The model under review builds one solid part; all positions refer to its coordinate system, in mm. Coordinates: 2 decimals unless noted, no trailing zeros. Write each loop counter-clockwise with the first axis right and the second up, starting at its lowest first coordinate (ties: lowest second). Pieces come first, ordered by that corner, then holes. Notation, with made-up numbers: (62, 21) - (91, 21) arc R13 ccw to (91, 43) - close; hole circle Ø10 at (-36, 63). An arc over 180 degrees is marked (long way). Put each result on its own line as item: value.
from build123d import *

# Parameters (mm, degrees)
F1_DEPTH = 25.4
F2_DEPTH = 25.4


with BuildPart() as f1:
    # F0 (on Top) → F1 (new body)
    with BuildSketch(Plane.XY):
        with BuildLine():
            ThreePointArc((22.225, -12.296722), (12.7, 0), (22.225, 12.296722))
            ThreePointArc((22.225, 12.296722), (-25.4, 0), (22.225, -12.296722))
        make_face()
        with BuildLine():
            ThreePointArc((22.225, -12.296722), (24.593444, -6.35), (25.4, 0))
            ThreePointArc((25.4, 0), (24.593444, 6.35), (22.225, 12.296722))
            ThreePointArc((22.225, 12.296722), (12.7, 0), (22.225, -12.296722))
        make_face()
    extrude(amount=F1_DEPTH)


with BuildPart() as f2:
    # F0 (on Top) → F2 (new body)
    with BuildSketch(Plane.XY):
        with BuildLine():
            ThreePointArc((22.225, 12.296722), (24.593444, 6.35), (25.4, 0))
            ThreePointArc((25.4, 0), (24.593444, -6.35), (22.225, -12.296722))
            ThreePointArc((22.225, -12.296722), (33.17713, -10.040232), (38.1, 0))
            ThreePointArc((38.1, 0), (33.17713, 10.040232), (22.225, 12.296722))
        make_face()
        with BuildLine():
            ThreePointArc((22.225, -12.296722), (24.593444, -6.35), (25.4, 0))
            ThreePointArc((25.4, 0), (24.593444, 6.35), (22.225, 12.296722))
            ThreePointArc((22.225, 12.296722), (12.7, 0), (22.225, -12.296722))
        make_face()
    extrude(amount=F2_DEPTH)

    # F3: intersect F1
    add(f1.part, mode=Mode.INTERSECT)


solid = f2.part
1. Consider section C-C on x = 24. State the section outline as (y, z) points.
Determined:
outline: (-8.32, 0) - (8.32, 0) - (8.32, 25.4) - (-8.32, 25.4) - close
2. For pin 1 Ø2 at (x, z) = (16.5, 5.5) entering from -Y; pin 2 Ø12 at (y, z) = (-8.5, 9) entering from -X; pin 3 Ø4 at (x, z) = (14.5, 22.5) entering from -Y, all flat-tipped, find the tip position at first contact; note any pin that passes through.
Determined:
pin 1: stops at y = -9.94
pin 2: stops at x = 12.95
pin 3: stops at y = -9.06
3. To check wall thickness, follow probe 1 along X at (y, z) = (-5, 18.25); probe 2 along Y at (x, z) = (16.5, 2.5); probe 3 along Y at (x, z) = (21, 17). State the ranges of each line that lie inside material, in increasing order.
Determined:
probe 1: x = 13.73 to 24.9
probe 2: y = -9.06 to 9.06
probe 3: y = -11.91 to 11.91
4. Consider section B-B on y = -9. State the section outline as (x, z) points, plus the area to 3 significant figures.
Determined:
outline: (16.44, 0) - (23.75, 0) - (23.75, 25.4) - (16.44, 25.4) - close
area: 186 mm^2
5. Consider section A-A on z = 14.25. State the section outline as (x, y) points (3 decimals), plus the area to 3 significant figures.
Determined:
outline: (22.225, -12.297) arc R25.4 ccw to (25.4, 0) arc R25.4 ccw to (22.225, 12.297) arc R12.7 ccw to start
area: 226 mm^2
